from build123d import *

# Parameters (mm, degrees)
F1_DEPTH = 3
F3_DEPTH = 8.7
F5_DEPTH = 6


with BuildPart() as f1:
    # F0 (on Front) → F1 (new body, symmetric)
    with BuildSketch(Plane.XZ):
        with BuildLine():
            Line((-8.9, 0), (-10.1, 0))
            Line((-10.1, 0), (-10.1, -2.6))
            Line((-10.1, -2.6), (-11.67, -2.6))
            Line((-11.67, -2.6), (-14.8, -2.6))
            Line((-14.8, -2.6), (-18.8, -2.6))
            Line((-18.8, -2.6), (-18.8, -4.7))
            Line((-18.8, -4.7), (0, -4.7))
            Line((0, -4.7), (4.7, -4.7))
            Line((4.7, -4.7), (4.7, 0))
            Line((4.7, 0), (3, 0))
            ThreePointArc((3, 0), (2.1213203436, -2.1213203436), (0, -3))
            ThreePointArc((0, -3), (-2.1213203436, -2.1213203436), (-3, 0))
            Line((-3, 0), (-4.7, 0))
            Line((-4.7, 0), (-4.7, -2.6))
            Line((-4.7, -2.6), (-8.9, -2.6))
            Line((-8.9, -2.6), (-8.9, 0))
        make_face()
    extrude(amount=F1_DEPTH, both=True)

    # F2 (on face) → F3 (cut, through all)
    with BuildSketch(Plane(origin=(-18.8, 0, 0), x_dir=(0, -1, 0), z_dir=(-1, 0, 0))):
        with BuildLine():
            Line((1.5, -2.6), (-1.5, -2.6))
            ThreePointArc((-1.5, -2.6), (0, -3.0019237886), (1.5, -2.6))
        make_face()
    extrude(amount=-F3_DEPTH, mode=Mode.SUBTRACT)

    # F4 (on face) → F5 (join, through all)
    with BuildSketch(Plane(origin=(0, 3, 0), x_dir=(-1, 0, 0), z_dir=(0, 1, 0))):
        with BuildLine():
            ThreePointArc((14.8, -2.6), (13.235, -1.9854598779), (11.67, -2.6))
            Line((11.67, -2.6), (11.67, -4.7))
            Line((11.67, -4.7), (14.8, -4.7))
            Line((14.8, -4.7), (14.8, -2.6))
        make_face()
    extrude(amount=-F5_DEPTH)

    # F6: F1 across plane


with BuildPart() as f1_1:
    add(f1.part)
    add(f1.part.mirror(Plane.XY))


solid = f1_1.part
Part model, mm, in its own coordinate system. A direction names the side the tool comes from. Give positions to 0.01 mm unless a question says otherwise; leave off trailing zeros. Order: outer loops, then holes, each group sorted by start corner. A loop starts at its lowest first (then second) coordinate and runs counter-clockwise, first axis right, second up. Notation, with made-up numbers: (76.25, 30.5) -> (92.25, 30.5) arc R10 cw to (92.25, 49.5) -> close; hole circle Ø11 at (69.25, 27). An arc over 180 degrees is marked (long way). Use one line per item in the form item = value.
(1) Saw through at A-A (x = -8.5). Write the cut outline in (y, z).
Solution:
outline = (-3, -4.7) -> (3, -4.7) -> (3, -2.6) -> (-3, -2.6) -> close; (-3, 2.6) -> (3, 2.6) -> (3, 4.7) -> (-3, 4.7) -> close
(2) Saw through at C-C (y = 1). Write the cut outline in (x, z) (3 decimals), then the cut area to 3 significant figures.
Solution:
outline = (-18.8, -4.7) -> (4.7, -4.7) -> (4.7, 4.7) -> (-18.8, 4.7) -> (-18.8, 2.83) -> (-14.8, 2.83) -> (-14.8, 2.6) arc R2.3 ccw to (-11.67, 2.6) -> (-11.67, 2.83) -> (-10.1, 2.83) -> (-10.1, -2.83) -> (-11.67, -2.83) -> (-11.67, -2.6) arc R2.3 ccw to (-14.8, -2.6) -> (-14.8, -2.83) -> (-18.8, -2.83) -> close; hole (-8.9, -2.6) -> (-4.7, -2.6) -> (-4.7, 2.6) -> (-8.9, 2.6) -> close; hole circle Ø6 at (0, 0)
area = 126 mm²
(3) Pull direction X, two halves, no side cores. Call faces 4 (the face through (-7, 0, -4.7)), 5 (the face through (-13.259, 0.042, -1.986)), 6 (the face through (-18.8, 0, -4)), 7 (the face through (-11, 2, 2.6)): +X half, -X half, draft (parallel to the pull), parting line (faces both ways), or undercut.
Solution:
face_4 = draft
face_5 = undercut
face_6 = -X half
face_7 = undercut
(4) Flat gauge pin, fed straight in: P1, Ø1, axis at y = 0.5, z = 1, coming from the -X side. Where does the tip first touch, or does it go through?
Solution:
P1 = -10.1
(5) Saw through at D-D (x = 0). Write the cut outline in (y, z), then the cut area to 3 significant figures.
Solution:
outline = (-3, -4.7) -> (3, -4.7) -> (3, -3) -> (-3, -3) -> close; (-3, 3) -> (3, 3) -> (3, 4.7) -> (-3, 4.7) -> close
area = 20.4 mm²
(6) Saw through at B-B (z = -2.25). Write the cut outline in (x, y).
Solution:
outline = (-14.31, -3) -> (-12.16, -3) -> (-12.16, 3) -> (-14.31, 3) -> close; (-10.1, -3) -> (-8.9, -3) -> (-8.9, 3) -> (-10.1, 3) -> close; (-4.7, -3) -> (-1.98, -3) -> (-1.98, 3) -> (-4.7, 3) -> close; (1.98, -3) -> (4.7, -3) -> (4.7, 3) -> (1.98, 3) -> close
(7) Drill centre lines: line 1 (X direction, y = -2.4, z = 1.5); line 2 (X direction, y = -1.6, z = -0.5); line 3 (Z direction, x = -8.25, y = 2.4). Where is each one in solid material? Low to high. Write a range as from..to.
Solution:
line_1 = -10.1..-8.9, -4.7..-2.6, 2.6..4.7
line_2 = -10.1..-8.9, -4.7..-2.96, 2.96..4.7
line_3 = -4.7..-2.6, 2.6..4.7
(8) Tool access for faces 1 (the face through (-17, 0, -3)), 2 (the face through (-17, 2, -2.6)), 3 (the face through (-11, -2, 2.6)): list every direction of +Z, -Z, +X, -X, +Y, -Y with a clear straight run to the whole face (end or side of a thin tool).
Solution:
face_1 = -X
face_2 = -X, +Y, -Y
face_3 = +Y, -Y
